Geometry: final body of the model. Coordinates: model frame, mm. A direction names the side the tool comes from. Give positions to 0.01 mm unless a question says otherwise; leave off trailing zeros. Write each loop counter-clockwise with the first axis right and the second up, starting at its lowest first coordinate (ties: lowest second). Pieces come first, ordered by that corner, then holes.
Q1. Section A-A (x = 4). Return the cut outline in (y, z).
Q2. Line query: line 1 (X direction, y = -17, z = 6); line 2 (X direction, y = -5.5, z = 21.75); line 3 (X direction, y = 15, z = 22). Output: solid intervals per line, ascending.
Q3. Section B-B (y = 20). Return the cut outline in (x, z), plus the area to 3 significant figures.
Q4. Pin query (flat end, axial travel): pin 1 Ø1 at (y, z) = (-12, 13) entering from +X; pin 2 Ø8 at (y, z) = (19, 3.5) entering from +X; pin 3 Ø1 at (x, z) = (-11.5, 13.5) entering from -Y; pin 4 Ø2 at (x, y) = (-14.5, -4) entering from -Z. Return the tip coordinate at first contact, or that it passes through.
Q5. Reachability of faces 1 (the flat face through (18, 9.702, 13)), 2 (the flat face through (-20, 10.43, 12)) from +Z, -Z, +X, -X, +Y, -Y: full face, straight path, thin tool, end or side. Return the list, or none.
Q6. Mould query, pull axis Y, two halves, no side actions, for faces 3 (the flat face through (-19, 9.702, 13)), 4 (the flat face through (20, 10.43, 12)), 5 (the flat face through (-7.3, 10.1, 0)). Classes: +Y half, -Y half, draft (parallel to the pull), parting line (faces both ways), or undercut.
from build123d import *

# Parameters (mm, degrees)
F1_DEPTH = 25.4
F2_SIZE  = 0.6604


with BuildPart() as f1:
    # F0 (on Top) → F1 (new body)
    with BuildSketch(Plane.XY):
        with BuildLine():
            Line((-12.2607089005, -3.9837458116), (-17.0759435824, -18.8035143197))
            ThreePointArc((-17.0759435824, -18.8035143197), (-16.7805039882, -19.0676345125), (-16.4809797049, -19.3271132859))
            Line((-16.4809797049, -19.3271132859), (-11.6417368792, -4.4334553087))
            Line((-11.6417368792, -4.4334553087), (-12.2607089005, -3.9837458116))
        make_face()
        with BuildLine():
            Line((-12.2607089005, -3.9837458116), (-12.0242826264, -3.2561005601))
            Line((-12.0242826264, -3.2561005601), (-24.6935848241, 5.9486862866))
            ThreePointArc((-24.6935848241, 5.9486862866), (-24.7833872632, 5.5627075929), (-24.8671569615, 5.1753748319))
            Line((-24.8671569615, 5.1753748319), (-12.2607089005, -3.9837458116))
        make_face()
        with BuildLine():
            Line((-12.606448061, -22.0507928947), (0, -12.8916722513))
            Line((0, -12.8916722513), (-0.6189720213, -12.4419627541))
            Line((-0.6189720213, -12.4419627541), (-13.2882742189, -21.6467496009))
            ThreePointArc((-13.2882742189, -21.6467496009), (-12.9489371469, -21.8514307716), (-12.606448061, -22.0507928947))
        make_face()
        with BuildLine():
            Line((-17.0759435824, -18.8035143197), (-18.8367259586, -24.2226452514))
            Line((-18.8367259586, -24.2226452514), (-18.4541802113, -25.4))
            Line((-18.4541802113, -25.4), (-16.4809797049, -19.3271132859))
            ThreePointArc((-16.4809797049, -19.3271132859), (-16.7805039882, -19.0676345125), (-17.0759435824, -18.8035143197))
        make_face()
        with BuildLine():
            Line((-18.4541802113, -25.4), (-17.2162361687, -25.4))
            Line((-17.2162361687, -25.4), (-12.606448061, -22.0507928947))
            ThreePointArc((-12.606448061, -22.0507928947), (-12.9489371469, -21.8514307716), (-13.2882742189, -21.6467496009))
            Line((-13.2882742189, -21.6467496009), (-18.4541802113, -25.4))
        make_face()
        Polygon((-18.8367259586, -24.2226452514), (-19.8382437272, -27.305), (-17.2162361687, -25.4), (-18.4541802113, -25.4), align=None)
        with BuildLine():
            ThreePointArc((-1.9732005064, 25.3232399144), (-2.3680385381, 25.2893731334), (-2.7623001448, 25.2493504453))
            Line((-2.7623001448, 25.2493504453), (-7.5775348267, 10.4295819372))
            Line((-7.5775348267, 10.4295819372), (-6.8124433322, 10.4295819372))
            Line((-6.8124433322, 10.4295819372), (-1.9732005064, 25.3232399144))
        make_face()
        with BuildLine():
            Line((6.8124433322, 10.4295819372), (7.5775348267, 10.4295819372))
            Line((7.5775348267, 10.4295819372), (2.7623001448, 25.2493504453))
            ThreePointArc((2.7623001448, 25.2493504453), (2.3680385381, 25.2893731334), (1.9732005064, 25.3232399144))
            Line((1.9732005064, 25.3232399144), (6.8124433322, 10.4295819372))
        make_face()
        with BuildLine():
            Line((12.2607089005, -3.9837458116), (24.8671569615, 5.1753748319))
            ThreePointArc((24.8671569615, 5.1753748319), (24.7833872632, 5.5627075929), (24.6935848241, 5.9486862866))
            Line((24.6935848241, 5.9486862866), (12.0242826264, -3.2561005601))
            Line((12.0242826264, -3.2561005601), (12.2607089005, -3.9837458116))
        make_face()
        with BuildLine():
            Line((17.0759435824, -18.8035143197), (12.2607089005, -3.9837458116))
            Line((12.2607089005, -3.9837458116), (11.6417368792, -4.4334553087))
            Line((11.6417368792, -4.4334553087), (16.4809797049, -19.3271132859))
            ThreePointArc((16.4809797049, -19.3271132859), (16.7805039882, -19.0676345125), (17.0759435824, -18.8035143197))
        make_face()
        Polygon((11.6417368792, -4.4334553087), (12.2607089005, -3.9837458116), (12.0242826264, -3.2561005601), (11.4053106051, -3.7058100573), align=None)
        with BuildLine():
            ThreePointArc((24.6935848241, 5.9486862866), (24.7833872632, 5.5627075929), (24.8671569615, 5.1753748319))
            Line((24.8671569615, 5.1753748319), (29.4769450692, 8.5245819372))
            Line((29.4769450692, 8.5245819372), (29.8594908165, 9.7019366858))
            Line((29.8594908165, 9.7019366858), (24.6935848241, 5.9486862866))
        make_face()
        Polygon((29.8594908165, 9.7019366858), (29.4769450692, 8.5245819372), (32.0989526277, 10.4295819372), (28.8579730479, 10.4295819372), align=None)
        with BuildLine():
            ThreePointArc((23.1599615849, 10.4295819372), (23.31985896, 10.0669845578), (23.4740798445, 9.7019366858))
            Line((23.4740798445, 9.7019366858), (29.8594908165, 9.7019366858))
            Line((29.8594908165, 9.7019366858), (28.8579730479, 10.4295819372))
            Line((28.8579730479, 10.4295819372), (23.1599615849, 10.4295819372))
        make_face()
        with BuildLine():
            Line((7.8139611007, 9.7019366858), (23.4740798445, 9.7019366858))
            ThreePointArc((23.4740798445, 9.7019366858), (23.31985896, 10.0669845578), (23.1599615849, 10.4295819372))
            Line((23.1599615849, 10.4295819372), (7.5775348267, 10.4295819372))
            Line((7.5775348267, 10.4295819372), (7.8139611007, 9.7019366858))
        make_face()
        Polygon((7.0488696062, 9.7019366858), (7.8139611007, 9.7019366858), (7.5775348267, 10.4295819372), (6.8124433322, 10.4295819372), align=None)
        with BuildLine():
            Line((-23.4740798445, 9.7019366858), (-7.8139611007, 9.7019366858))
            Line((-7.8139611007, 9.7019366858), (-7.5775348267, 10.4295819372))
            Line((-7.5775348267, 10.4295819372), (-23.1599615849, 10.4295819372))
            ThreePointArc((-23.1599615849, 10.4295819372), (-23.31985896, 10.0669845578), (-23.4740798445, 9.7019366858))
        make_face()
        with BuildLine():
            Line((-23.1599615849, 10.4295819372), (-28.8579730479, 10.4295819372))
            Line((-28.8579730479, 10.4295819372), (-29.8594908165, 9.7019366858))
            Line((-29.8594908165, 9.7019366858), (-23.4740798445, 9.7019366858))
            ThreePointArc((-23.4740798445, 9.7019366858), (-23.31985896, 10.0669845578), (-23.1599615849, 10.4295819372))
        make_face()
        Polygon((-28.8579730479, 10.4295819372), (-32.0989526277, 10.4295819372), (-29.4769450692, 8.5245819372), (-29.8594908165, 9.7019366858), align=None)
        with BuildLine():
            Line((-29.8594908165, 9.7019366858), (-29.4769450692, 8.5245819372))
            Line((-29.4769450692, 8.5245819372), (-24.8671569615, 5.1753748319))
            ThreePointArc((-24.8671569615, 5.1753748319), (-24.7833872632, 5.5627075929), (-24.6935848241, 5.9486862866))
            Line((-24.6935848241, 5.9486862866), (-29.8594908165, 9.7019366858))
        make_face()
        Polygon((-7.8139611007, 9.7019366858), (-7.0488696062, 9.7019366858), (-6.8124433322, 10.4295819372), (-7.5775348267, 10.4295819372), align=None)
        Polygon((0, -12.8916722513), (0.6189720213, -12.4419627541), (0, -11.992253257), (-0.6189720213, -12.4419627541), align=None)
        with BuildLine():
            Line((13.2882742189, -21.6467496009), (0.6189720213, -12.4419627541))
            Line((0.6189720213, -12.4419627541), (0, -12.8916722513))
            Line((0, -12.8916722513), (12.606448061, -22.0507928947))
            ThreePointArc((12.606448061, -22.0507928947), (12.9489371469, -21.8514307716), (13.2882742189, -21.6467496009))
        make_face()
        with BuildLine():
            Line((17.2162361687, -25.4), (18.4541802113, -25.4))
            Line((18.4541802113, -25.4), (13.2882742189, -21.6467496009))
            ThreePointArc((13.2882742189, -21.6467496009), (12.9489371469, -21.8514307716), (12.606448061, -22.0507928947))
            Line((12.606448061, -22.0507928947), (17.2162361687, -25.4))
        make_face()
        with BuildLine():
            Line((18.8367259586, -24.2226452514), (17.0759435824, -18.8035143197))
            ThreePointArc((17.0759435824, -18.8035143197), (16.7805039882, -19.0676345125), (16.4809797049, -19.3271132859))
            Line((16.4809797049, -19.3271132859), (18.4541802113, -25.4))
            Line((18.4541802113, -25.4), (18.8367259586, -24.2226452514))
        make_face()
        Polygon((19.8382437272, -27.305), (18.8367259586, -24.2226452514), (18.4541802113, -25.4), (17.2162361687, -25.4), align=None)
        with BuildLine():
            Line((0, 31.3961266285), (-1.0015177686, 30.6684813771))
            Line((-1.0015177686, 30.6684813771), (-2.7623001448, 25.2493504453))
            ThreePointArc((-2.7623001448, 25.2493504453), (-2.3680385381, 25.2893731334), (-1.9732005064, 25.3232399144))
            Line((-1.9732005064, 25.3232399144), (0, 31.3961266285))
        make_face()
        with BuildLine():
            Line((2.7623001448, 25.2493504453), (1.0015177686, 30.6684813771))
            Line((1.0015177686, 30.6684813771), (0, 31.3961266285))
            Line((0, 31.3961266285), (1.9732005064, 25.3232399144))
            ThreePointArc((1.9732005064, 25.3232399144), (2.3680385381, 25.2893731334), (2.7623001448, 25.2493504453))
        make_face()
        Polygon((1.0015177686, 30.6684813771), (0, 33.7508361256), (-1.0015177686, 30.6684813771), (0, 31.3961266285), align=None)
        Polygon((-11.6417368792, -4.4334553087), (-11.4053106051, -3.7058100573), (-12.0242826264, -3.2561005601), (-12.2607089005, -3.9837458116), align=None)
    extrude(amount=F1_DEPTH)

    # F2
    f2_edges = [f1.edges().sort_by_distance(p)[0] for p in [
        (-19.838244, 10.429582, 25.4),
        (-22.179831, 3.222918, 25.4),
        (-16.049476, -15.644373, 25.4),
        (-9.919122, -20.098336, 25.4),
        (9.919122, -20.098336, 25.4),
        (16.049476, -15.644373, 25.4),
        (22.179831, 3.222918, 25.4),
        (19.838244, 10.429582, 25.4),
        (3.788767, 22.090209, 25.4),
        (-3.788767, 22.090209, 25.4),
    ]]
    chamfer(f2_edges, length=F2_SIZE)


solid = f1.part
Computed:
1. outline: (-15.8, 0) - (-14.9, 0) - (-14.9, 25.4) - (-14.98, 25.4) - (-15.8, 24.74) - close; (19.09, 0) - (21.44, 0) - (21.44, 24.74) - (19.3, 25.4) - (19.09, 25.4) - close
2. line 1: x = -16.49 to -15.72, -6.89 to -5.65, 5.65 to 6.89, 15.72 to 16.49
2. line 2: x = -12.75 to -11.99, 11.99 to 12.75
2. line 3: x = -6.09 to -5.33, 5.33 to 6.09
3. outline: (-4.47, 0) - (-3.7, 0) - (-3.7, 25.4) - (-3.77, 25.4) - (-4.47, 24.74) - close; (3.7, 0) - (4.47, 0) - (4.47, 24.74) - (3.77, 25.4) - (3.7, 25.4) - close
3. area: 38.4 mm2
4. pin 1: stops at x = 15.03
4. pin 2: stops at x = 6.09
4. pin 3: stops at y = -21.61
4. pin 4: passes through
5. face 1: +Z, -Z
5. face 2: +Z, -Z, -X, +Y
6. face 3: undercut
6. face 4: +Y half
6. face 5: draft
